Here's how the part is built. I have some questions about the finished solid (model axes, mm). Coordinates: 2 decimals unless noted, no trailing zeros. Loops run counter-clockwise (first coordinate to the right, second up) from the corner with the lowest first, then second, coordinate; pieces in that order, holes last. Notation, with made-up numbers: (74, 45) -> (83, 45) arc R24 cw to (83, 55) -> close; hole circle Ø6 at (32, 47.5). An arc over 180 degrees is marked (long way). Answer as a JSON object with one key per item and string values. Group by question number.
1) I need wall thicknesses on probe 1 along Z at (x, y) = (48.5, 0.75); probe 2 along Y at (x, z) = (460.5, 20.5) (3 decimals); probe 3 along X at (y, z) = (-7, -28) (3 decimals). Which ranges of each line are inside material? Lowest first, please. Write a range as [from, to].
2) I'm going to push flat-ended pins straight in: pin 1 (10 mm diameter, centred on x = 490, z = 28, fed in from +Y); pin 2 (3 mm diameter, centred on x = -169, y = 4, fed in from -Z); pin 3 (6 mm diameter, centred on y = 0.5, z = -15, fed in from +X) (3 decimals). Where does each tip first touch, or does it pass through?
3) I want a section at A-A (x = -507.5). Write out the boundary of the cut face in (y, z) (3 decimals), then the cut area to 3 significant figures.
4) I want a section at B-B (y = 3.5). Write out the boundary of the cut face in (x, z) (3 decimals), then the cut area to 3 significant figures.
```python
from build123d import *

# Parameters (mm, degrees)
F1_DEPTH      = 1219.2
F1_DEPTH_BACK = 1219.2
F3_DEPTH      = 63.501


with BuildPart() as f1:
    # F0 (on Right) → F1 (new body, two sides)
    with BuildSketch(Plane.YZ) as f1_sk:
        Polygon((0, 31.75), (-9.525, 31.75), (-9.525, -31.75), (0, -31.75), (0, -19.05), (9.525, -19.05), (9.525, 19.05), (0, 19.05), align=None)
    extrude(amount=F1_DEPTH)
    extrude(f1_sk.sketch, amount=-F1_DEPTH_BACK)

    # F2 (on face) → F3 (cut, through all)
    with BuildSketch(Plane.XY.offset(31.75)):
        Polygon((-1219.2, 0), (-1209.675, 0), (-1200.15, 9.525), (-1219.2, 9.525), align=None)
        Polygon((-1219.2, 0), (-1219.2, -9.525), (-1209.675, 0), align=None)
        Polygon((1200.15, 9.525), (1209.675, 0), (1219.2, 0), (1219.2, 9.525), align=None)
        Polygon((1209.675, 0), (1219.2, -9.525), (1219.2, 0), align=None)
    extrude(amount=-F3_DEPTH, mode=Mode.SUBTRACT)


solid = f1.part
```
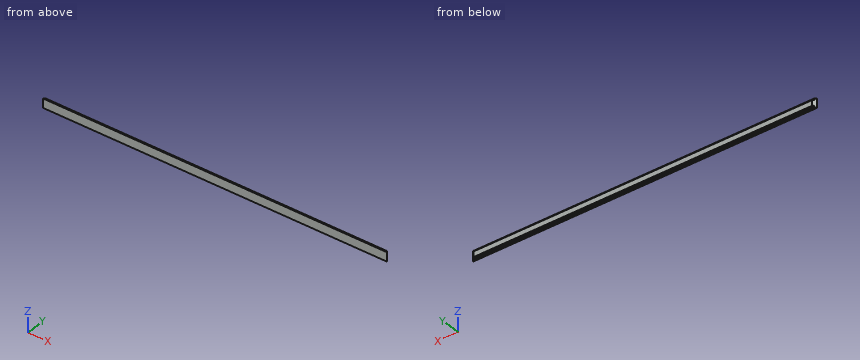
Determined:
{
 "1": {"probe 1": "[-19.05, 19.05]", "probe 2": "[-9.525, 0]", "probe 3": "[-1216.675, 1216.675]"},
 "2": {"pin 1": "y = 0", "pin 2": "z = -19.05", "pin 3": "x = 1212.175"},
 "3": {"outline": "(-9.525, -31.75) -> (0, -31.75) -> (0, -19.05) -> (9.525, -19.05) -> (9.525, 19.05) -> (0, 19.05) -> (0, 31.75) -> (-9.525, 31.75) -> close", "area": "968 mm^2"},
 "4": {"outline": "(-1206.175, -19.05) -> (1206.175, -19.05) -> (1206.175, 19.05) -> (-1206.175, 19.05) -> close", "area": "91,900 mm^2"}
}
